Autodesk Inventor part; units mm, degrees
ref_plane "YZ Plane" through (0, 0, 0) normal (1, 0, 0) x (0, 1, 0)
ref_plane "XZ Plane" through (0, 0, 0) normal (0, 1, 0) x (-1, 0, 0)
ref_plane "XY Plane" through (0, 0, 0) normal (0, 0, 1) x (1, 0, 0)
sketch "Sketch1" plane through (0, 0, 0) normal (0, 1, 0) x (-1, 0, 0)
  line L0 (0, 0) -> (301.4, 0)
  line L1 (301.4, 0) -> (42.4, -259)
  line L2 (42.4, -259) -> (0, -301.4)
  line L3 (0, -301.4) -> (0, 0)
  line L4 (301.4, 0) -> (286.4, 0)
  line L5 (286.4, 0) -> (286.4, 3.2)
  line L6 (286.4, 3.2) -> (246.4, 3.2)
  line L7 (246.4, 3.2) -> (246.4, 0)
  line L8 (0, 0) -> (15, 0)
  line L9 (15, 0) -> (15, 3.2)
  line L10 (15, 3.2) -> (55, 3.2)
  line L11 (55, 3.2) -> (55, 0)
  line L12 (55, 0) -> (15, 0)
  dimension "d0" = 301.4
  dimension "d1" = 45
  dimension "d2" = 15
  dimension "d3" = 3.2
  dimension "d4" = 40
  dimension "d5" = 15
  dimension "d6" = 40
extrude "Extrusion1" add sketch "Sketch1" along normal blind 3.175
properties part number "Trebuchet V1 - Truss Support"
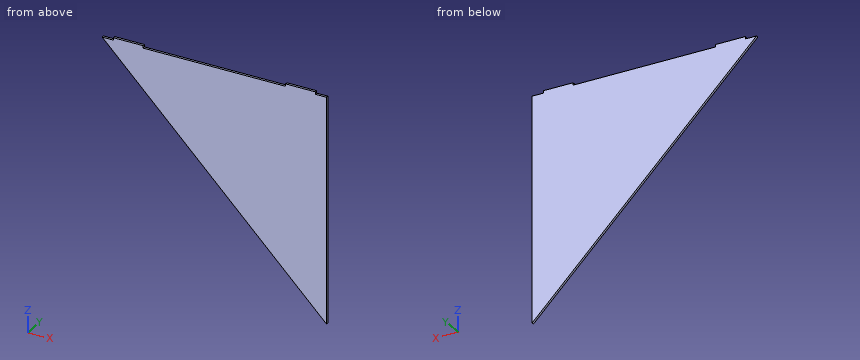
Source: CAD feature listing. Evaluate the final solid. Frame: model axes, mm. Give positions to 0.01 mm unless a question says otherwise; leave off trailing zeros. Write each loop counter-clockwise with the first axis right and the second up, starting at its lowest first coordinate (ties: lowest second). Pieces come first, ordered by that corner, then holes. Notation, with made-up numbers: M -25.5,-22 L -10.5,-22 A20 cw -10.5,-4 Z; hole C 62.25,55 d9. An arc over 180 degrees is marked long. Return JSON: item names as keys, results as strings. Group by question number.
1) Material intervals for line 1 along X through (y, z) = (1.35, -33); line 2 along X through (y, z) = (0.6, -256); line 3 along Z through (x, y) = (-56.5, 2.35), sorted ascending. Write a range as [from, to].
2) Cut plane A-A, the plane y = 2.25. Output: boundary loops of the cut face in (x, z).
3) Cut plane C-C, the plane z = -136.5. Output: boundary loops of the cut face in (x, y) (3 decimals).
4) Pin query (flat end, axial travel): P1, Ø4, axis at x = -70, z = -162, coming from the -Y side; P2, Ø1.6, axis at x = -293.5, y = 1, coming from the +Z side; P3, Ø1, axis at y = 1.5, z = 2, coming from the -X side. Return the tip coordinate at first contact, or that it passes through.
5) Cut plane B-B, the plane x = -112.5. Output: boundary loops of the cut face in (y, z) (3 decimals).
Recorded:
{
 "1": {"line 1": "x = [-268.4, 0]", "line 2": "x = [-45.4, 0]", "line 3": "z = [-244.9, 0]"},
 "2": {"outline": "M -301.4,0 L 0,-301.4 L 0,0 L -15,0 L -15,3.2 L -55,3.2 L -55,0 L -246.4,0 L -246.4,3.2 L -286.4,3.2 L -286.4,0 Z"},
 "3": {"outline": "M -164.9,0 L 0,0 L 0,3.175 L -164.9,3.175 Z"},
 "4": {"P1": "stops at y = 0", "P2": "stops at z = 0", "P3": "stops at x = -286.4"},
 "5": {"outline": "M 0,-188.9 L 3.175,-188.9 L 3.175,0 L 0,0 Z"}
}
